Autodesk Inventor part; units mm, degrees
ref_plane "YZ Plane" through (0, 0, 0) normal (1, 0, 0) x (0, 1, 0)
ref_plane "XZ Plane" through (0, 0, 0) normal (0, 1, 0) x (-1, 0, 0)
ref_plane "XY Plane" through (0, 0, 0) normal (0, 0, 1) x (1, 0, 0)
sketch "Skizze1" plane through (0, 0, 0) normal (0, 0, 1) x (1, 0, 0)
  line L0 (-50, 9) -> (-50, -9) construction
  line L1 (50, 9) -> (50, -9) construction
  line L2 (-50, -9) -> (-50, 9)
  line L3 (-50, 9) -> (-25.1982, 9)
  line L4 (25.1982, 9) -> (50, 9)
  line L5 (50, -9) -> (25.1982, -9)
  line L6 (-25.1982, -9) -> (-50, -9)
  line L7 (50, 9) -> (29.5255, 5.3146) construction
  arc A0 (25.1982, 9) -> (-25.1982, 9) centre (0, 0) ccw
  arc A1 (-25.1982, -9) -> (25.1982, -9) centre (0, 0) ccw
  line L8 (50, -12.5) -> (50, -9) construction
  line L9 (50, 9) -> (50, 12.5) construction
  line L10 (50, 9) -> (50, -9)
  point P0 (0, 0)
  dimension "d13" = 100
  dimension "d14" = 18
extrude "Extrusion1" add sketch "Skizze1" along normal blind 3
sketch "Skizze3" plane through (0, 0, 0) normal (0, 0, -1) x (-1, 0, 0)
  line L0 (50, -12.5) -> (50, 12.5) construction
  line L1 (50, 12.5) -> (27.2718, 12.5) construction
  arc A0 (27.2718, 12.5) -> (-27.2718, 12.5) centre (0, 0) ccw construction
  line L2 (-27.2718, 12.5) -> (-50, 12.5) construction
  line L3 (-50, 12.5) -> (-50, -12.5) construction
  line L4 (-50, -12.5) -> (-27.2718, -12.5) construction
  arc A1 (-27.2718, -12.5) -> (27.2718, -12.5) centre (0, 0) ccw construction
  line L5 (27.2718, -12.5) -> (50, -12.5) construction
  line L6 (50, 9) -> (50, -9)
  line L7 (50, -9) -> (25.1982, -9)
  arc A2 (-25.1982, -9) -> (25.1982, -9) centre (0, 0) ccw
  line L8 (-25.1982, -9) -> (-50, -9)
  line L9 (-50, -9) -> (-50, 9)
  line L10 (-50, 9) -> (-25.1982, 9)
  arc A3 (25.1982, 9) -> (-25.1982, 9) centre (0, 0) ccw
  line L11 (25.1982, 9) -> (50, 9)
  line L12 (-26.5702, 11) -> (-52, 11)
  line L13 (-52, 11) -> (-52, -11)
  line L14 (-52, -11) -> (-26.5702, -11)
  arc A4 (-26.5702, -11) -> (26.5702, -11) centre (0, 0) ccw
  line L15 (26.5702, -11) -> (52, -11)
  line L16 (52, -11) -> (52, 11)
  line L17 (52, 11) -> (26.5702, 11)
  arc A5 (26.5702, 11) -> (-26.5702, 11) centre (0, 0) ccw
  dimension "d15" = 2
extrude "Extrusion3" add sketch "Skizze3" against normal up to surface (3 mm away)
properties part number "Emblem"
Can you work these out from the model? Positions are in its coordinate system, mm. A direction names the side the tool comes from. Round coordinates to 2 decimals unless told otherwise and drop trailing zeros. Loops run counter-clockwise (first coordinate to the right, second up) from the corner with the lowest first, then second, coordinate; pieces in that order, holes last. Notation, with made-up numbers: (49, 67) -> (53, 67) arc R18 cw to (53, 96) -> close; hole circle Ø4 at (-34.5, 41.5). An arc over 180 degrees is marked (long way). Answer in a Markdown table with one row per item.
Item 1: If I drill on probe 1 along Y at (x, z) = (35, 2.2); probe 2 along Y at (x, z) = (0, 1.85); probe 3 along X at (y, z) = (18.5, 1.15), over which ranges is the centre line in solid material (lowest first)?
Answer block:
| item | result |
|---|---|
| probe 1 | -11 to 11 |
| probe 2 | -28.76 to 28.76 |
| probe 3 | -22.02 to 22.02 |
Item 2: Suppose I cut it at A-A, the plane z = 2.25. List the corners of the cut face in (x, y) for me, plus the area to 3 significant figures.
Answer block:
| item | result |
|---|---|
| outline | (-52, -11) -> (-26.57, -11) arc R28.76 ccw to (26.57, -11) -> (52, -11) -> (52, 11) -> (26.57, 11) arc R28.76 ccw to (-26.57, 11) -> (-52, 11) -> close |
| area | 3,650 mm² |
Item 3: On a 3-axis mill with a long thin cutter (end or side, diameter ignored), from which of +Z, -Z, +X, -X, +Y, -Y can I reach the whole of each face in a straight line? I mean faces 1 (the flat face through (-39, -11, 1)), 2 (the flat face through (39, 11, 1)), 3 (the flat face through (39, -11, 1)), 4 (the flat face through (-1, 0, 0)), 5 (the flat face through (-39, 11, 1)). Say none if no direction works.
Answer block:
| item | result |
|---|---|
| face 1 | +Z, -Z, -X, -Y |
| face 2 | +Z, -Z, +X, +Y |
| face 3 | +Z, -Z, +X, -Y |
| face 4 | -Z, +X, -X, +Y, -Y |
| face 5 | +Z, -Z, -X, +Y |
Item 4: Will these pins go through, and if not, where does the flat tip stop? P1, Ø0.9, axis at x = -34, z = 1, coming from the +Y side; P2, Ø1, axis at y = -20.5, z = 0.5, coming from the -X side; P3, Ø1.5, axis at x = -2.5, z = 2, coming from the +Y side.
Answer block:
| item | result |
|---|---|
| P1 | y = 11 |
| P2 | x = -20.66 |
| P3 | y = 28.7 |
Item 5: Suppose I cut it at B-B, the plane x = -17.5. List the corners of the cut face in (y, z) for me.
Answer block:
| item | result |
|---|---|
| outline | (-22.82, 0) -> (22.82, 0) -> (22.82, 3) -> (-22.82, 3) -> close |
Item 6: Suppose I cut it at C-C, the plane y = -24. List the corners of the cut face in (x, z) for me, plus the area to 3 significant figures.
Answer block:
| item | result |
|---|---|
| outline | (-15.84, 0) -> (15.84, 0) -> (15.84, 3) -> (-15.84, 3) -> close |
| area | 95.1 mm² |
